Part print with two shaded views. Sizes in mm from the minimum x, y, z corner. Coordinates: 2 decimals unless noted, no trailing zeros. Order: outer loops, then holes, each group sorted by start corner. A loop starts at its lowest first (then second) coordinate and runs counter-clockwise, first axis right, second up. Notation, with made-up numbers: (-0.5, -11.75) - (35.5, -11.75) arc R29 ccw to (35.5, 23.25) - close; hole circle Ø7 at (-23.75, 22.25). An arc over 180 degrees is marked (long way). Return JSON: item names as keys, results as strings.
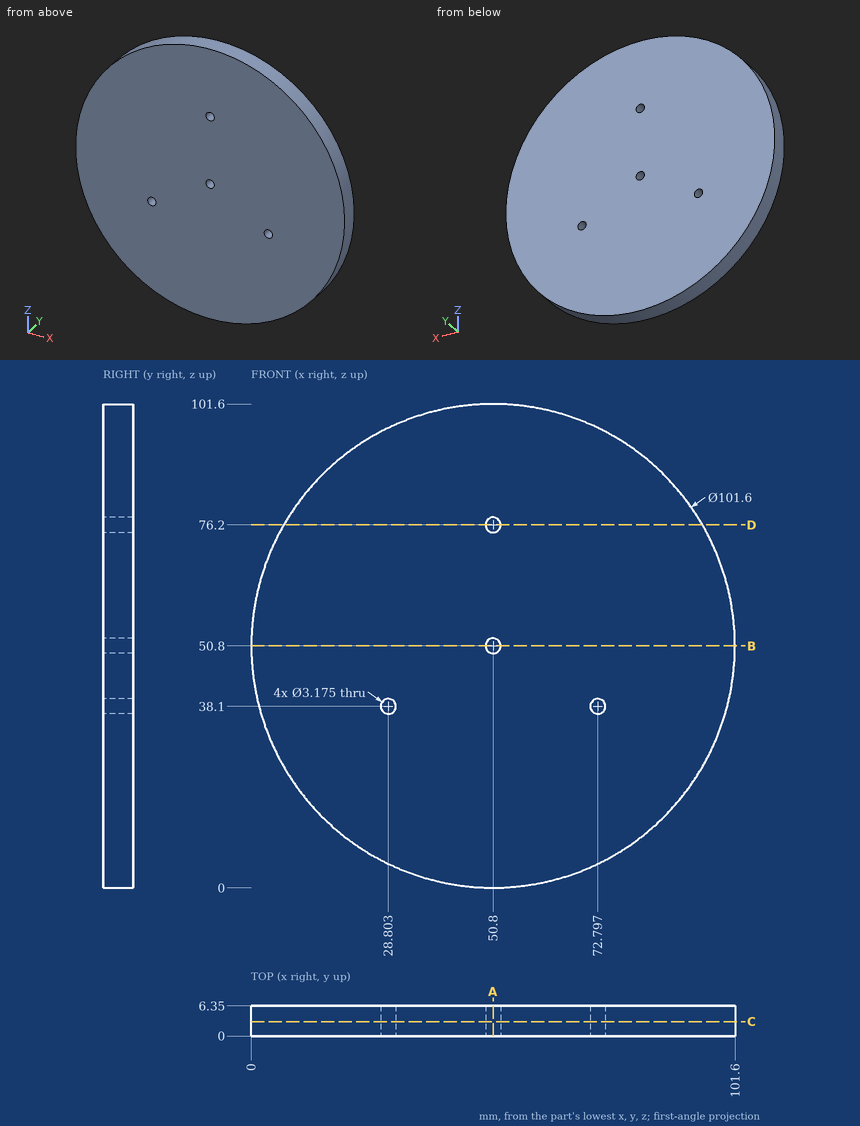
Item 1: Band-saw the part on C-C, the plane y = 3. List the corners of the cut face in (x, z) (1 decimal).
Findings below:
{"outline": "circle Ø101.6 at (50.8, 50.8); hole circle Ø3.2 at (28.8, 38.1); hole circle Ø3.2 at (50.8, 50.8); hole circle Ø3.2 at (50.8, 76.2); hole circle Ø3.2 at (72.8, 38.1)"}
Item 2: Band-saw the part on D-D, the plane z = 76.2. List the corners of the cut face in (x, y).
Findings below:
{"outline": "(6.81, 0) - (49.21, 0) - (49.21, 6.35) - (6.81, 6.35) - close; (52.39, 0) - (94.79, 0) - (94.79, 6.35) - (52.39, 6.35) - close"}
Item 3: Band-saw the part on A-A, the plane x = 50.8. List the corners of the cut face in (y, z), then the cut area to 3 significant figures.
Findings below:
{"outline": "(0, 0) - (6.35, 0) - (6.35, 49.21) - (0, 49.21) - close; (0, 52.39) - (6.35, 52.39) - (6.35, 74.61) - (0, 74.61) - close; (0, 77.79) - (6.35, 77.79) - (6.35, 101.6) - (0, 101.6) - close", "area": "605 mm²"}
Item 4: Drop flat-ended pins along their axis: P1, Ø3.5, axis at x = 50.8, z = 50.8, coming from the +Y side; P2, Ø3, axis at y = 2, z = 42.5, coming from the +X side; P3, Ø3, axis at x = 64.5, y = 5, coming from the +Z side; P4, Ø2.5, axis at x = 72.8, z = 38.1, coming from the +Y side. Give the stop position or say it passes through.
Findings below:
{"P1": "stops at y = 6.35", "P2": "stops at x = 101.14", "P3": "stops at z = 100.11", "P4": "passes through"}
Item 5: Band-saw the part on B-B, the plane z = 50.8. List the corners of the cut face in (x, y).
Findings below:
{"outline": "(0, 0) - (49.21, 0) - (49.21, 6.35) - (0, 6.35) - close; (52.39, 0) - (101.6, 0) - (101.6, 6.35) - (52.39, 6.35) - close"}
Item 6: Wall check: L1, parallel to Z at x = 50.8, y = 4.5; L2, parallel to X at y = 1.5, z = 38.1; L3, parallel to X at y = 1.5, z = 76.2. Give the ranges that are in metal, low to high. Write a range as [from, to].
Findings below:
{"L1": "z = [0, 49.21], [52.39, 74.61], [77.79, 101.6]", "L2": "x = [1.61, 27.22], [30.39, 71.21], [74.38, 99.99]", "L3": "x = [6.81, 49.21], [52.39, 94.79]"}
